Check sheet for the drawn part. Datum: minimum x, y, z corner. Units: mm. Give positions to 0.01 mm unless a question says otherwise; leave off trailing zeros. Order: outer loops, then holes, each group sorted by start corner. A loop starts at its lowest first (then second) coordinate and runs counter-clockwise, first axis right, second up.
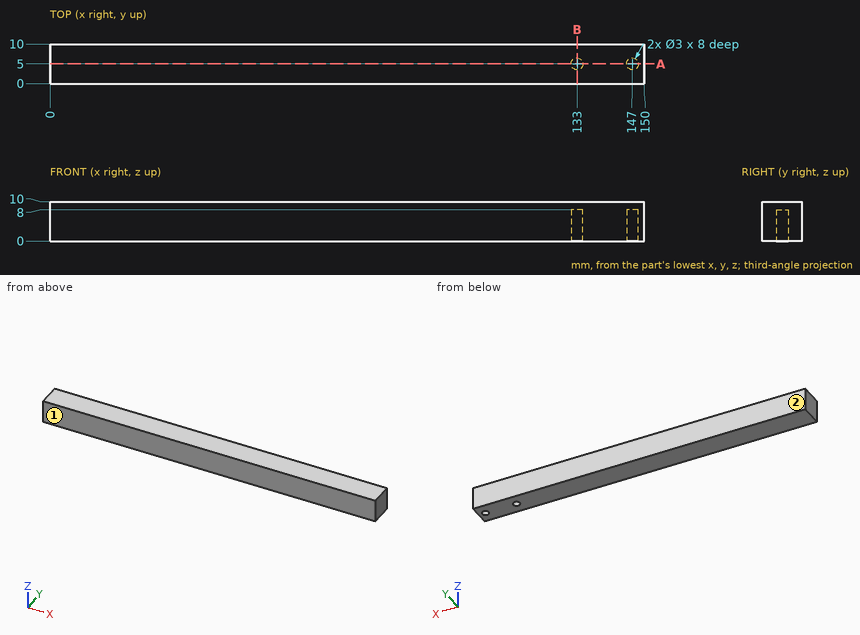
Q1. Material ranges on line 1 (X direction, y = 5, z = 4); line 2 (Y direction, x = 147, z = 3.5); line 3 (X direction, y = 6, z = 5.75), recorded low to high.
Q2. Sectioned sample at A-A, the plane y = 5. Record the cut outline in (x, z).
Q3. Sectioned sample at B-B, the plane x = 133. Record the cut outline in (y, z).
Q4. Draft check along Y on the marked faces 1 and 2. Enter one of: pulls with the +Y half, pulls with the -Y half, needs draft (parallel to the pull), parting line crosses it, or undercut.
Q5. Go/stop test with flat-tipped pins: P1, Ø2.5, axis at x = 147, y = 5, coming from the -Z side; P2, Ø2.5, axis at x = 146.5, y = 5, coming from the -Z side. Record where each tip stops, or that it passes through.
Filled in:
1. line 1: x = 0 to 131.5, 134.5 to 145.5, 148.5 to 150
1. line 2: y = 0 to 3.5, 6.5 to 10
1. line 3: x = 0 to 131.88, 134.12 to 145.88, 148.12 to 150
2. outline: (0, 0) - (131.5, 0) - (131.5, 8) - (134.5, 8) - (134.5, 0) - (145.5, 0) - (145.5, 8) - (148.5, 8) - (148.5, 0) - (150, 0) - (150, 10) - (0, 10) - close
3. outline: (0, 0) - (3.5, 0) - (3.5, 8) - (6.5, 8) - (6.5, 0) - (10, 0) - (10, 10) - (0, 10) - close
4. face 1: pulls with the -Y half
4. face 2: pulls with the +Y half
5. P1: stops at z = 8
5. P2: stops at z = 0
